```python
from build123d import *

# Parameters (mm, degrees)
F0_W        = 35
F0_H        = 30
F1_DEPTH    = 30.5
F2_T        = -1
F4_D        = 15
F4_DEPTH    = 12
F4_TIP      = 4.5064546427
F5_T1_DEPTH = 45.2867319519
F6_T1_DEPTH = 45.2867319519


# Not quite as in the source:
# - a fillet or chamfer that OpenCascade refuses, or shapes differently, is made with other operations: its cross-section is extruded or revolved along the edge and cut away or added


with BuildPart() as f1:
    # F0 (on Top) → F1 (new body)
    with BuildSketch(Plane.XY):
        with Locations((17.5, 15)):
            Rectangle(F0_W, F0_H)
    extrude(amount=F1_DEPTH)

    # F2
    f2_openings = [f1.faces().sort_by_distance(p)[0] for p in [
        (17.5, 15, 30.5),
    ]]
    offset(amount=F2_T, openings=f2_openings)

    # F4
    with Locations(Plane(origin=(0, 0, 0), x_dir=(0, 1, 0), z_dir=(-1, 0, 0))):
        with Locations((15, -15)):
            Hole(F4_D / 2, depth=F4_DEPTH)
            with Locations((0, 0, -(F4_DEPTH + F4_TIP / 2))):  # 118° drill point
                Cone(0, F4_D / 2, F4_TIP, mode=Mode.SUBTRACT)

    # F5: chamfer of 2 on 1 edges, made by hand

    # F5_s2 → F5_t1 (cut)
    with BuildSketch(Plane.YZ.offset(-5.1433659759)):
        Polygon((2, 30.5), (0, 28.5), (0, 30.5), align=None)
    extrude(amount=F5_T1_DEPTH, mode=Mode.SUBTRACT)

    # F6: chamfer of 2 on 1 edges, made by hand

    # F6_s2 → F6_t1 (cut)
    with BuildSketch(Plane.YZ.offset(-5.1433659759)):
        Polygon((28, 30.5), (30, 28.5), (30, 30.5), align=None)
    extrude(amount=F6_T1_DEPTH, mode=Mode.SUBTRACT)


solid = f1.part
```
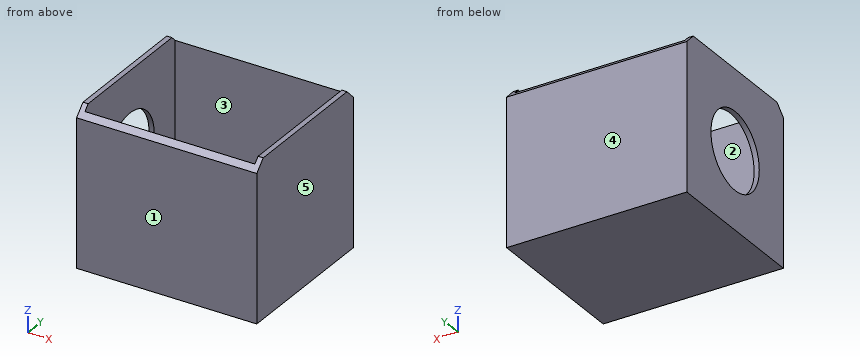
Input: part model. Units: mm. Frame: model coordinates. Face numbers are marked on the shaded views. A direction names the side the tool comes from. Coordinates: 2 decimals unless noted, no trailing zeros. Write each loop counter-clockwise with the first axis right and the second up, starting at its lowest first coordinate (ties: lowest second). Pieces come first, ordered by that corner, then holes. Notation, with made-up numbers: (-23, 17.5) - (-8, 17.5) arc R30 cw to (-8, 53.5) - close; hole circle Ø6 at (-35, 79). An arc over 180 degrees is marked (long way). Put each result on its own line as item: value. Start each with the question number.
1) Reachability of the marked faces 1 and 2 from +Z, -Z, +X, -X, +Y, -Y: full face, straight path, thin tool, end or side. Return the list, or none.
2) Cut plane D-D (z = 15). Return the cut outline in (x, y).
3) Ray query, L1, parallel to X at y = 10.25, z = 23; L2, parallel to Y at x = 29.5, z = 18.5; L3, parallel to Z at x = 0.55, y = 15. Return the intervals inside material, ascending.
4) Contact query for flat-ended pins moving along their axis: pin 1 (2 mm diameter, centred on x = 5, z = 19, fed in from -Y); pin 2 (2 mm diameter, centred on x = 23.5, y = 8.5, fed in from +Z). Output: stop coordinate, or through.
5) Mould query, pull axis Y, two halves, no side actions, for the marked faces 3, 4 and 5. Classes: pulls with the +Y half, pulls with the -Y half, needs draft (parallel to the pull), parting line crosses it, or undercut.
6) Cut plane A-A (y = 15). Return the cut outline in (x, z).
7) Cut plane C-C (y = 2.5). Return the cut outline in (x, z), plus the area to 3 significant figures.
8) Cut plane B-B (z = 5). Return the cut outline in (x, y), plus the area to 3 significant figures.
Resolved:
1. face 1: +Z, -Z, +X, -X, -Y
1. face 2: +Z
2. outline: (0, 0) - (35, 0) - (35, 30) - (0, 30) - (0, 22.5) - (1, 22.5) - (1, 29) - (34, 29) - (34, 1) - (1, 1) - (1, 7.5) - (0, 7.5) - close
3. L1: x = 0 to 1, 34 to 35
3. L2: y = 0 to 1, 29 to 30
3. L3: z = 0 to 7.5, 22.5 to 30.5
4. pin 1: stops at y = 0
4. pin 2: stops at z = 1
5. face 3: undercut
5. face 4: pulls with the +Y half
5. face 5: needs draft
6. outline: (0, 0) - (35, 0) - (35, 30.5) - (34, 30.5) - (34, 1) - (1, 1) - (1, 7.5) - (0, 7.5) - close; (0, 22.5) - (1, 22.5) - (1, 30.5) - (0, 30.5) - close
7. outline: (0, 0) - (35, 0) - (35, 30.5) - (34, 30.5) - (34, 1) - (1, 1) - (1, 30.5) - (0, 30.5) - close
7. area: 94.0 mm2
8. outline: (0, 0) - (35, 0) - (35, 30) - (0, 30) - close; hole (1, 1) - (34, 1) - (34, 29) - (1, 29) - close
8. area: 126 mm2
